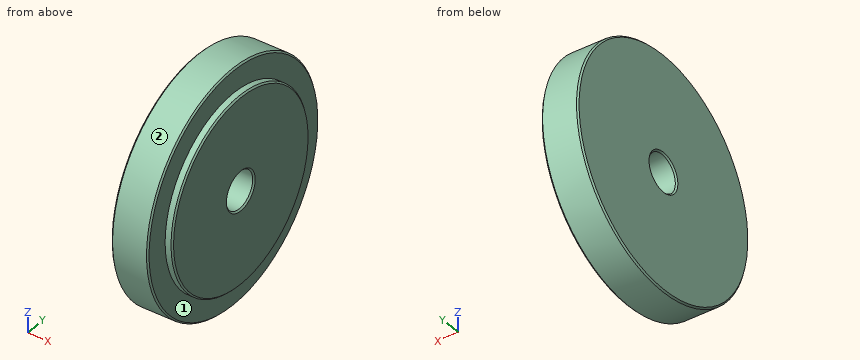
from build123d import *

# Parameters (mm, degrees)
F2_R     = 12.5
F3_DEPTH = 40
F4_SIZE  = 1


with BuildPart() as f1:
    # F0 (on Front) → F1 (revolve)
    with BuildSketch(Plane.XZ):
        Polygon((25, 80), (0, 80), (0, 0), (30, 0), (30, 64), (25, 64), align=None)
    revolve(axis=Axis((15, 0, 0), (-1, 0, 0)))

    # F2 (on face) → F3 (cut)
    with BuildSketch(Plane.YZ.offset(30)):
        Circle(F2_R)
    extrude(amount=-F3_DEPTH, mode=Mode.SUBTRACT)

    # F4
    f4_edges = [f1.edges().sort_by_distance(p)[0] for p in [
        (30, 0, -64),
        (30, -12.5, 0),
        (25, 0, -80),
        (0, 0, -80),
        (0, -12.5, 0),
    ]]
    chamfer(f4_edges, length=F4_SIZE)


solid = f1.part
Build history of the part. All positions in model axes, mm. Face numbers are marked on the shaded views. A direction names the side the tool comes from. Round coordinates to 2 decimals unless told otherwise and drop trailing zeros. Loops run counter-clockwise (first coordinate to the right, second up) from the corner with the lowest first, then second, coordinate; pieces in that order, holes last. Notation, with made-up numbers: (-38.5, -23.5) -> (-30.5, -23.5) arc R17 cw to (-30.5, -7.5) -> close; hole circle Ø5 at (27.5, 57). An arc over 180 degrees is marked (long way). Answer in a Markdown table with one row per item.
Item 1: Pin check, flat tips, straight feed: pin 1 (8 mm diameter, centred on x = 16.5, y = -36.5, fed in from +Z); pin 2 (1 mm diameter, centred on x = 5.5, z = 59.5, fed in from +Y); pin 3 (5 mm diameter, centred on x = 12.5, z = -19.5, fed in from -Y); pin 4 (15 mm diameter, centred on y = 0, z = 0, fed in from +X). Stop position of each tip, or through.
Answers below:
| item | result |
|---|---|
| pin 1 | stops at z = 73.1 |
| pin 2 | stops at y = 54.03 |
| pin 3 | stops at y = -78.17 |
| pin 4 | passes through |
Item 2: Drill centre lines: L1, parallel to Z at x = 13.75, y = -0.5; L2, parallel to X at y = -55, z = -42; L3, parallel to Z at x = 19, y = -2 (3 decimals). Where is each one in solid material? Low to high. Write a range as [from, to].
Answers below:
| item | result |
|---|---|
| L1 | z = [-80, -12.49], [12.49, 80] |
| L2 | x = [0, 25] |
| L3 | z = [-79.975, -12.339], [12.339, 79.975] |
Item 3: Saw through at C-C (x = 9.25). Write the cut outline in (y, z).
Answers below:
| item | result |
|---|---|
| outline | circle Ø160 at (0, 0); hole circle Ø25 at (0, 0) |
Item 4: Which spindle directions (+Z, -Z, +X, -X, +Y, -Y) get a long thin tool onto all of the face, cutting with end or side? Do the marked faces 1 and 2. Say none if no direction does.
Answers below:
| item | result |
|---|---|
| face 1 | +X |
| face 2 | +X, -X |
Item 5: Saw through at A-A (z = 0). Write the cut outline in (x, y), and give its area (4 significant figures).
Answers below:
| item | result |
|---|---|
| outline | (0, -79) -> (1, -80) -> (24, -80) -> (25, -79) -> (25, -64) -> (29, -64) -> (30, -63) -> (30, -13.5) -> (29, -12.5) -> (1, -12.5) -> (0, -13.5) -> close; (0, 13.5) -> (1, 12.5) -> (29, 12.5) -> (30, 13.5) -> (30, 63) -> (29, 64) -> (25, 64) -> (25, 79) -> (24, 80) -> (1, 80) -> (0, 79) -> close |
| area | 3,885 mm² |
